Part model, mm, in its own coordinate system. A direction names the side the tool comes from. Give positions to 0.01 mm unless a question says otherwise; leave off trailing zeros. Order: outer loops, then holes, each group sorted by start corner. A loop starts at its lowest first (then second) coordinate and runs counter-clockwise, first axis right, second up.
1. Slice it at A-A on x = 30.78. List the corners of the cut face in (y, z).
2. Which spindle directions (+Z, -Z, +X, -X, +Y, -Y) get a long thin tool onto all of the face, cutting with end or side? Do faces 4 (the flat face through (30, 14.75, -1)), 5 (the flat face through (27, 11, -7.109)), 6 (the cylindrical face through (32.688, 15.601, 9.86)). Say none if no direction does.
3. Slice it at D-D on x = 22.5. List the corners of the cut face in (y, z), and give its area (3 significant figures).
4. Mould opens along Y. For faces 1 (the flat face through (31, 23, 0)), 2 (the flat face through (30, 15.25, -1)), 3 (the flat face through (31, 0, -5)) say: +Y half, -Y half, draft (parallel to the pull), parting line (faces both ways), or undercut.
5. Probe line 1 (Z direction, x = 28.15, y = 15); line 2 (Y direction, x = 30.78, z = -47); line 3 (X direction, y = 5, z = -6). List the from-to ranges inside material, lowest first.
6. Drop flat-ended pins along their axis: pin 1 Ø3 at (x, y) = (21.5, 11) entering from -Z; pin 2 Ø4.5 at (x, y) = (28, 19) entering from +Z; pin 3 Ø8 at (x, y) = (60, 11) entering from +Z. Give the stop position or say it passes through.
7. Slice it at B-B on y = 5. List the corners of the cut face in (x, z).
8. Slice it at C-C on z = -16.5. List the corners of the cut face in (x, y), and give its area (3 significant figures).
from build123d import *

# Parameters (mm, degrees)
BOSS_EXTRUDE1_DEPTH      = 30
SKETCH3_R                = 4.5
SKETCH3_R_2              = 2.5
BOSS_EXTRUDE3_DEPTH      = 50
CUT_EXTRUDE2_REACH       = 71.06
SKETCH7_R                = 1.5
SKETCH8_R                = 2
BOSS_EXTRUDE6_DEPTH      = 20
SKETCH9_W                = 5
SKETCH9_H                = 0.5
CUT_EXTRUDE14_DEPTH      = 15
SKETCH11_W               = 5
SKETCH11_H               = 0.5
CUT_EXTRUDE16_DEPTH      = 1
CUT_EXTRUDE16_DEPTH_BACK = 4
FILLET1_R                = 0.5
SKETCH10_W               = 5
SKETCH10_H               = 0.5
CUT_EXTRUDE15_DEPTH      = 107.779594


with BuildPart() as part:
    # Sketch1 → Boss-Extrude1 (new body)
    with BuildSketch(Plane(origin=(0, 0, 0), x_dir=(1, 0, 0), z_dir=(0, 1, 0))):
        with BuildLine():
            Line((15.281403332, 7.10934213), (46.278596668, 7.10934213))
            ThreePointArc((46.278596668, 7.10934213), (60.283738602, 11.932467089), (69.06, 0))
            ThreePointArc((69.06, 0), (61.56, 7.5), (54.06, 0))
            Line((54.06, 0), (7.5, 0))
            ThreePointArc((7.5, 0), (0, 7.5), (-7.5, 0))
            ThreePointArc((-7.5, 0), (1.276261398, 11.932467089), (15.281403332, 7.10934213))
        make_face()
    extrude(amount=BOSS_EXTRUDE1_DEPTH)

    # Sketch3 → Boss-Extrude3 (add)
    with BuildSketch(Plane(origin=(0, 0, -7.10934213), x_dir=(-1, 0, 0), z_dir=(0, 0, -1))):
        with Locations((-30.78, 15)):
            Circle(SKETCH3_R)
        with Locations((-30.78, 15)):
            Circle(SKETCH3_R_2, mode=Mode.SUBTRACT)
    extrude(amount=BOSS_EXTRUDE3_DEPTH)

    # Sketch7 → Cut-Extrude2 (cut, up to next)
    with BuildSketch(Plane(origin=(0, 0, 0), x_dir=(0, 0, -1), z_dir=(1, 0, 0)), mode=Mode.PRIVATE) as cut_extrude2_sk1:
        with Locations((53.042344304, 15)):
            Circle(SKETCH7_R)
    cut_extrude2_tool1 = extrude(cut_extrude2_sk1.sketch, amount=CUT_EXTRUDE2_REACH, mode=Mode.PRIVATE) & part.part
    add(cut_extrude2_tool1.solids().sort_by_distance((0, 15, -53.042344))[0], mode=Mode.SUBTRACT)

    # Sketch8 → Boss-Extrude6 (add)
    with BuildSketch(Plane.XY):
        with Locations((30.78, 15)):
            Circle(SKETCH8_R)
    extrude(amount=BOSS_EXTRUDE6_DEPTH)

    # Sketch9 → Cut-Extrude14 (cut)
    with BuildSketch(Plane(origin=(0, 0, 0), x_dir=(0, 0, -1), z_dir=(1, 0, 0))):
        with Locations((0, 15.381990369)):
            Rectangle(SKETCH9_W, SKETCH9_H)
    extrude(amount=-CUT_EXTRUDE14_DEPTH, mode=Mode.SUBTRACT)

    # Sketch11 → Cut-Extrude16 (cut, two sides)
    with BuildSketch(Plane(origin=(68.252070678, 0, 0), x_dir=(0, 0, -1), z_dir=(-1, 0, 0))) as cut_extrude16_sk:
        with Locations((0, -15)):
            Rectangle(SKETCH11_W, SKETCH11_H)
    extrude(amount=CUT_EXTRUDE16_DEPTH, mode=Mode.SUBTRACT)
    extrude(cut_extrude16_sk.sketch, amount=-CUT_EXTRUDE16_DEPTH_BACK, mode=Mode.SUBTRACT)

    # Fillet1
    fillet1_edges = [part.edges().sort_by_distance(p)[0] for p in [
        (35.28, 15, -7.10934213),
    ]]
    fillet(fillet1_edges, radius=FILLET1_R)

    # Sketch10 → Cut-Extrude15 (cut)
    with BuildSketch(Plane(origin=(0, 0, 0), x_dir=(0, 0, -1), z_dir=(1, 0, 0))):
        with Locations((0, 15)):
            Rectangle(SKETCH10_W, SKETCH10_H)
    extrude(amount=CUT_EXTRUDE15_DEPTH, mode=Mode.SUBTRACT)


solid = part.part
Data:
1. outline: (0, -7.11) - (10, -7.11) arc R0.5 cw to (10.5, -7.61) - (10.5, -57.11) - (12.5, -57.11) - (12.5, -7.11) - (17.5, -7.11) - (17.5, -57.11) - (19.5, -57.11) - (19.5, -7.61) arc R0.5 cw to (20, -7.11) - (30, -7.11) - (30, 0) - (17, 0) - (17, 20) - (13, 20) - (13, 0) - (0, 0) - close; hole (14.75, -2.5) - (15.25, -2.5) - (15.25, 2.5) - (14.75, 2.5) - close
2. face 4: +X
2. face 5: -Z
2. face 6: +Z
3. outline: (0, -7.11) - (30, -7.11) - (30, 0) - (15.25, 0) - (15.25, -2.5) - (14.75, -2.5) - (14.75, 0) - (0, 0) - close
3. area: 212 mm2
4. face 1: draft
4. face 2: undercut
4. face 3: -Y half
5. line 1: z = -57.11 to -54.54, -51.54 to -2.5
5. line 2: y = 10.5 to 12.5, 17.5 to 19.5
5. line 3: x = -5.97 to -4.5, 4.5 to 57.06, 66.06 to 67.53
6. pin 1: stops at z = -7.11
6. pin 2: stops at z = 0
6. pin 3: stops at z = -5.03
7. outline: (-7.5, 0) arc R12.5 ccw to (15.28, -7.11) - (46.28, -7.11) arc R12.5 ccw to (69.06, 0) arc R7.5 cw to (54.06, 0) - (7.5, 0) arc R7.5 cw to start
8. outline: circle Ø9 at (30.78, 15); hole circle Ø5 at (30.78, 15)
8. area: 44.0 mm2
